Here's how the part is built. I have some questions about the finished solid (model axes, mm). Face numbers are marked on the shaded views. A direction names the side the tool comes from. Give positions to 0.01 mm unless a question says otherwise; leave off trailing zeros. Order: outer loops, then holes, each group sorted by start corner. A loop starts at its lowest first (then second) coordinate and runs counter-clockwise, first axis right, second up. Notation, with made-up numbers: M -19.75,0.25 L 21.25,0.25 A15 cw 21.25,29.25 Z; hole C 17,36.5 d7. An arc over 180 degrees is marked long. Use CSV: the item, a comma, the result in double quotes. Start each with the question number.
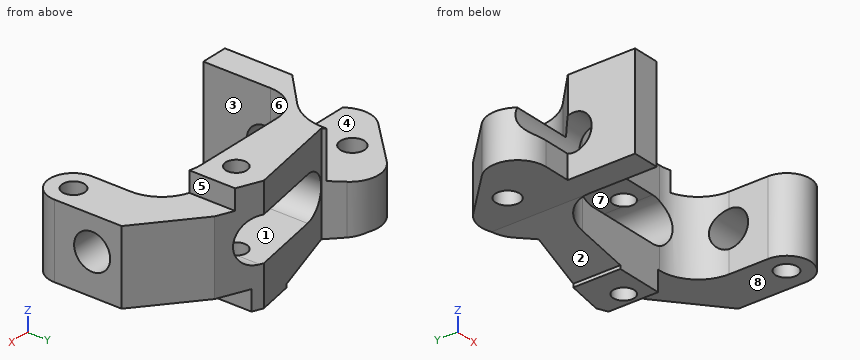
```python
from build123d import *

# Parameters (mm, degrees)
F1_DEPTH  = 17
F2_R      = 5
F4_DEPTH  = 25
F7_DEPTH  = 7
F8_R      = 1.6228798791
F8_R_2    = 1.552456108
F8_R_3    = 1.7623350299
F10_DEPTH = 25
F9_R      = 2.6750370967
F11_DEPTH = 37.3


with BuildPart() as f1:
    # F0 (on Top) → F1 (new body)
    with BuildSketch(Plane.XY):
        with BuildLine():
            Line((-4, 0), (0, 0))
            Line((0, 0), (0, 15))
            Line((0, 15), (19.25, 15))
            ThreePointArc((19.25, 15), (23.3158639918, 13.3158639918), (25, 9.25))
            Line((25, 9.25), (25, 3.5))
            ThreePointArc((25, 3.5), (28.5, 0), (32, 3.5))
            Line((32, 3.5), (32, 13.5))
            Line((32, 13.5), (23.5, 20.4821200219))
            Line((23.5, 20.4821200219), (17.5, 22.9821200219))
            Line((17.5, 22.9821200219), (3.725022686, 20.4821200219))
            Line((3.725022686, 20.4821200219), (2.0120524503, 22.9449909018))
            ThreePointArc((2.0120524503, 22.9449909018), (-1.159330371, 24.7860054935), (-4.6061857342, 23.5345296327))
            Line((-4.6061857342, 23.5345296327), (-10.9701467649, 17.170568602))
            ThreePointArc((-10.9701467649, 17.170568602), (-11.8806837632, 12.5929899911), (-8, 10))
            Line((-8, 10), (-4, 10))
            Line((-4, 10), (-4, 0))
        make_face()
    extrude(amount=F1_DEPTH)

    # F2
    f2_edges = [f1.edges().sort_by_distance(p)[0] for p in [
        (0, 15, 8.5),
    ]]
    fillet(f2_edges, radius=F2_R)

    # F3 (on Front) → F4 (intersect)
    with BuildSketch(Plane.XZ):
        Polygon((12, 0), (19, 0), (19, 3), (32, 3), (32, 14), (21, 14), (21, 17), (-13, 17), (-13, 3), (0, 3), (12, 0.5), align=None)
        with BuildLine():
            Line((18, 6), (7, 6))
            ThreePointArc((7, 6), (3.75, 9.25), (7, 12.5))
            Line((7, 12.5), (18, 12.5))
            ThreePointArc((18, 12.5), (21.25, 9.25), (18, 6))
        make_face(mode=Mode.SUBTRACT)
    extrude(amount=-F4_DEPTH, mode=Mode.INTERSECT)

    # F6 (on offset) → F7 (cut)
    with BuildSketch(Plane.XY.offset(17)):
        with BuildLine():
            Line((3.1616305932, 22.3574396223), (2.5333629455, 31.5121971071))
            Line((2.5333629455, 31.5121971071), (-19.064229839, 31.5121971071))
            Line((-19.064229839, 31.5121971071), (-10.1016564295, 4.1825510561))
            Line((-10.1016564295, 4.1825510561), (0.9379045805, 14.6835977212))
            ThreePointArc((0.9379045805, 14.6835977212), (3.08761934, 18.2197699763), (3.1616305932, 22.3574396223))
        make_face()
    extrude(amount=-F7_DEPTH, mode=Mode.SUBTRACT)

    # F8 (on Top) → F10 (cut)
    with BuildSketch(Plane.XY):
        with Locations((28.5243559629, 3.5737901926)):
            Circle(F8_R)
        with Locations((16.8598778546, 18.3908306062)):
            Circle(F8_R_2)
        with Locations((-5.050426349, 18.0755741894)):
            Circle(F8_R_3)
    extrude(amount=F10_DEPTH, mode=Mode.SUBTRACT)

    # F9 (on Right) → F11 (cut, symmetric)
    with BuildSketch(Plane.YZ):
        with Locations((9.1190673411, 9.0270899236)):
            Circle(F9_R)
    extrude(amount=F11_DEPTH, both=True, mode=Mode.SUBTRACT)


solid = f1.part
```
Q1. Imagine slicing it at B-B, the plane y = 8.5. Please give me the cut outline in (x, z), then the cut area to 3 significant figures.
Q2. Imagine slicing it at D-D, the plane x = 8. Please give me the cut outline in (y, z).
Q3. Imagine slicing it at C-C, the plane z = 14.75. Please give me the cut outline in (x, y), then the cut area to 3 significant figures.
Q4. I need wall thicknesses on line 1 (X direction, y = 3.5, z = 3.5); line 2 (Z direction, x = 17, y = 20.75); line 3 (X direction, y = 19.25, z = 9.25). Which ranges of each line are inside material? Lowest first, please. Write a range as [from, to].
Q5. We'd pull the mould along Z, two halves only. Please class the marked faces 1, 2 and 3: pulls with the +Z half, pulls with the -Z half, needs draft (parallel to the pull), parting line crosses it, or undercut.
Q6. For the marked faces 4, 5, 6, 7 and 8, which set-ups out of +Z, -Z, +X, -X, +Y, -Y let a thin tool reach every point of the face, with its end or its side?
Q7. For P1, Ø8, axis at y = 6.5, z = 13.5, coming from the -X side; P2, Ø1.5, axis at x = -7.5, y = 19.5, coming from the -Z side; P3, Ø7, axis at y = 9.12, z = 9.03, coming from the +X side; P4, Ø1.1, axis at x = -6.5, z = 4.5, coming from the -Y side, each with a flat end and sliding along its axis, tell me the tip position at first contact or that it passes through.
Q8. Imagine slicing it at A-A, the plane x = 28.5. Please give me the cut outline in (y, z) (3 decimals), then the cut area to 3 significant figures.
Reply:
1,outline,"M -4,3 L 0,3 L 0,6.42 L -4,6.42 Z; M -4,11.63 L 0,11.63 L 0,17 L -4,17 Z; M 25,3 L 32,3 L 32,6.42 L 25,6.42 Z; M 25,11.63 L 32,11.63 L 32,14 L 25,14 Z"
1,area,"75.7 mm^2"
2,outline,"M 15,1.33 L 21.26,1.33 L 21.26,6 L 15,6 Z; M 15,12.5 L 21.26,12.5 L 21.26,17 L 15,17 Z"
3,outline,"M -4,0 L 0,0 L 0,10 A5 cw 5,15 L 19.25,15 A5.75 cw 21,14.73 L 21,21.52 L 17.5,22.98 L 3.73,20.48 L 3.38,20.98 A7.92 cw 0.94,14.68 L -4,9.99 Z; hole C 16.86,18.39 d3.1"
3,area,"168 mm^2"
4,line 1,"x = [-4, 0], [25, 26.9], [30.15, 32]"
4,line 2,"z = [0, 6], [12.5, 17]"
4,line 3,"x = [-8.89, -6.36], [-3.74, 3.75], [21.25, 25]"
5,face 1,"undercut"
5,face 2,"pulls with the -Z half"
5,face 3,"needs draft"
6,face 4,"+Z, -X, +Y"
6,face 5,"+Z, +X, +Y, -Y"
6,face 6,"+Z, -Z, -Y"
6,face 7,"+Y, -Y"
6,face 8,"-Z, +X, +Y, -Y"
7,P1,"stops at x = -4"
7,P2,"stops at z = 3"
7,P3,"stops at x = 32"
7,P4,"stops at y = 10"
8,outline,"M 0,3 L 1.951,3 L 1.951,14 L 0,14 Z; M 5.196,3 L 16.375,3 L 16.375,14 L 5.196,14 Z; hole C 9.119,9.027 d5.35"
8,area,"122 mm^2"
